Could you check a few things on this drawing? It's one solid part, dimensions in mm from its lowest x, y, z. Give positions to 0.01 mm unless a question says otherwise; leave off trailing zeros. Loops run counter-clockwise (first coordinate to the right, second up) from the corner with the lowest first, then second, coordinate; pieces in that order, holes last.
Q1. Suppose I cut it at B-B (z = 36). List the corners of the cut face in (x, y) for me.
Q2. I need wall thicknesses on probe 1 along Z at (x, y) = (95.7, 2.1); probe 2 along X at (y, z) = (1.3, 31); probe 3 along Z at (x, y) = (155.7, 1.35). Which ranges of each line are inside material? Lowest first, please.
Q3. I'm going to push flat-ended pins straight in: P1, Ø1.2, axis at x = 35.7, z = 105, coming from the +Y side; P2, Ø1.7, axis at y = 2.5, z = 94, coming from the +X side; P3, Ø3, axis at y = 2, z = 88, coming from the -X side. Where does each tip first touch, or does it pass through?
Q4. Suppose I cut it at A-A (x = 62.5). List the corners of the cut face in (y, z) for me, and give its area (4 significant figures).
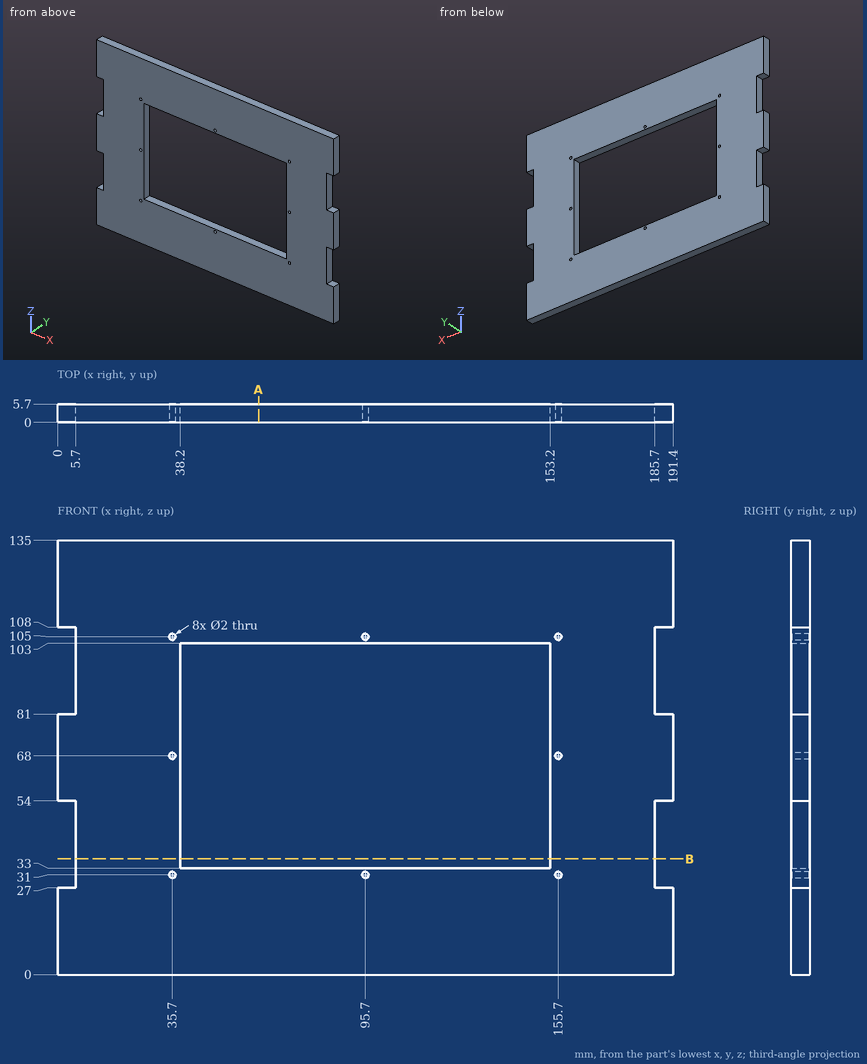
Solutions:
1. outline: (5.7, 0) - (38.2, 0) - (38.2, 5.7) - (5.7, 5.7) - close; (153.2, 0) - (185.7, 0) - (185.7, 5.7) - (153.2, 5.7) - close
2. probe 1: z = 0 to 30, 32 to 33, 103 to 104, 106 to 135
2. probe 2: x = 5.7 to 34.7, 36.7 to 94.7, 96.7 to 154.7, 156.7 to 185.7
2. probe 3: z = 0 to 30, 32 to 67, 69 to 104, 106 to 135
3. P1: passes through
3. P2: stops at x = 185.7
3. P3: stops at x = 5.7
4. outline: (0, 0) - (5.7, 0) - (5.7, 33) - (0, 33) - close; (0, 103) - (5.7, 103) - (5.7, 135) - (0, 135) - close
4. area: 370.5 mm2
